Here's how the part is built. I have some questions about the finished solid (model axes, mm). A direction names the side the tool comes from. Coordinates: 2 decimals unless noted, no trailing zeros. Write each loop counter-clockwise with the first axis right and the second up, starting at its lowest first coordinate (ties: lowest second). Pieces come first, ordered by that corner, then holes. Notation, with made-up numbers: (35.25, 4.5) - (70.25, 4.5) arc R27 cw to (70.25, 41.5) - close; hole circle Ø6 at (-13.5, 63). An arc over 180 degrees is marked (long way). Answer in a Markdown table with one row per item. Add a question column.
Item 1: Imagine slicing it at C-C (z = 6.75). Please give me the cut outline in (x, y).
Item 2: Imagine slicing it at D-D (x = -4.5). Please give me the cut outline in (y, z), plus the area to 3 significant figures.
Item 3: Which directions (+Z, -Z, +X, -X, +Y, -Y) give clear straight access to the entire face, cutting with the end or side of a thin tool? Please do faces 1 (the face through (-5.5, 0, 1)), 2 (the face through (-0.3, 4.5, 0)), 3 (the face through (32, 0, 6)).
Item 4: If I drill on probe 1 along Y at (x, z) = (-15.9, 3); probe 2 along Y at (x, z) = (0, 2); probe 3 along Z at (x, y) = (4.5, 3.25), over which ranges is the centre line in solid material (lowest first)? Write a range as from..to.
Item 5: I'm going to push flat-ended pins straight in: pin 1 (3 mm diameter, centred on x = 17, y = 0.5, fed in from +Z); pin 2 (1 mm diameter, centred on y = 4, z = 3.5, fed in from -X). Where does each tip first touch, or does it pass through?
Item 6: Imagine slicing it at A-A (y = 0). State how many separate pieces and enclosed holes the cut face has, plus the area to 3 significant figures.
Item 7: We'd pull the mould along Y, two halves only. Please class faces 4 (the face through (-34.5, -0.1, 3)), 5 (the face through (-29, 0, 7.55)), 6 (the face through (5.5, 0, 1)), 7 (the face through (0, -5, 2)): +Y half, -Y half, draft (parallel to the pull), parting line (faces both ways), or undercut.
Item 8: Imagine slicing it at B-B (x = 15.9). Please give me the cut outline in (y, z).
Autodesk Inventor part; units mm, degrees
ref_plane "YZ Plane" through (0, 0, 0) normal (1, 0, 0) x (0, 1, 0)
ref_plane "XZ Plane" through (0, 0, 0) normal (0, 1, 0) x (-1, 0, 0)
ref_plane "XY Plane" through (0, 0, 0) normal (0, 0, 1) x (1, 0, 0)
sketch "Sketch1" plane through (0, 0, 0) normal (0, 0, 1) x (1, 0, 0)
  circle A0 centre (0, 0) radius 3
  circle A1 centre (0, 0) radius 5 construction
  circle A2 centre (-29.5, 0) radius 2.5
  circle A3 centre (29.5, 0) radius 2.5
  line L0 (-29.5, 0) -> (29.5, 0) construction
  arc A4 (-29.5, 5) -> (-29.5, -5) centre (-29.5, 0) ccw
  arc A5 (29.5, -5) -> (29.5, 5) centre (29.5, 0) ccw
  line L1 (-29.5, 5) -> (29.5, 5)
  line L2 (29.5, -5) -> (-29.5, -5)
  dimension "d0" = 6
  dimension "d1" = 10
  dimension "d2" = 5
  dimension "d3" = 5
  dimension "d4" = 29.5
  dimension "d5" = 29.5
  dimension "d6" = 2.5
  dimension "d7" = 2.5
extrude "Extrusion1" add sketch "Sketch1" along normal blind 4.05
sketch "Sketch2" plane through (0, 0, 0) normal (0, 0, -1) x (-1, 0, 0)
  line L0 (-5.5, -4) -> (5.5, -4)
  line L1 (5.5, -4) -> (5.5, 4)
  line L2 (5.5, 4) -> (-5.5, 4)
  line L3 (-5.5, 4) -> (-5.5, -4)
  line L4 (-5.5, -4) -> (5.5, 4) construction
  line L5 (5.5, -4) -> (-5.5, 4) construction
  line L6 (-29.5, 5) -> (29.5, 5)
  point P0 (0, 0)
  dimension "d10" = 8
  dimension "d11" = 11
extrude "Extrusion2" cut sketch "Sketch2" against normal blind 1.3
sketch "Sketch3" plane through (0, 0, 0) normal (0, 0, -1) x (-1, 0, 0)
  circle A0 centre (-29.5, 0) radius 2.5
  circle A1 centre (29.5, 0) radius 2.5
  point P0 (0, 0)
extrude "Extrusion3" add sketch "Sketch3" against normal blind 7.55
sketch "Sketch4" plane through (-29.5, 5, 0) normal (0, 1, 0) x (1, 0, 0)
  line L0 (64, 0) -> (64, -4.05)
  line L1 (64, -2) -> (64, 0)
  line L2 (59, 0) -> (64, 0)
  line L3 (64, 0) -> (48.5, 0)
  arc A0 (48.5, 0) -> (64, -2) centre (62.5699, 47.9795) ccw
  line L4 (59, 0) -> (0, 0)
  line L5 (29.5, 0) -> (29.5, -4.05)
  line L6 (59, -4.05) -> (0, -4.05)
  line L7 (-5, -2) -> (-5, 0)
  line L8 (0, 0) -> (-5, 0)
  line L9 (-5, 0) -> (10.5, 0)
  arc A1 (-5, -2) -> (10.5, 0) centre (-3.5699, 47.9795) ccw
  dimension "d16" = 19
  dimension "d17" = 2
  dimension "d18" = 50
extrude "Extrusion4" cut sketch "Sketch4" against normal through all
sketch "Sketch5" plane through (0, 0, 0) normal (0, 0, -1) x (-1, 0, 0)
  circle A0 centre (15.9, 0) radius 0.9
  circle A1 centre (-15.9, 0) radius 0.9
  line L0 (15.9, 0) -> (-15.9, 0)
  point P0 (0, 0)
  dimension "d21" = 1.8
  dimension "d22" = 1.8
  dimension "d24" = 15.9
extrude "Extrusion5" cut sketch "Sketch5" against normal through all
equation "\"d3\" = d2"
properties part number "gripper_mechanism1"
Here are the results:
| question | item | result |
|---|---|---|
| 1 | outline | circle Ø5 at (-29.5, 0); circle Ø5 at (29.5, 0) |
| 2 | outline | (-5, 0) - (-4, 0) - (-4, 1.3) - (4, 1.3) - (4, 0) - (5, 0) - (5, 4.05) - (-5, 4.05) - close |
| 2 | area | 30.1 mm2 |
| 3 | face 1 | -Z |
| 3 | face 2 | -Z, +X, -X, +Y, -Y |
| 3 | face 3 | +Z |
| 4 | probe 1 | y = -5..-0.9, 0.9..5 |
| 4 | probe 2 | y = -5..-3, 3..5 |
| 4 | probe 3 | z = 1.3..4.05 |
| 5 | pin 1 | stops at z = 4.05 |
| 5 | pin 2 | stops at x = -33.07 |
| 6 | separate pieces | 4 |
| 6 | enclosed holes | 0 |
| 6 | area | 225 mm2 |
| 7 | face 4 | parting line |
| 7 | face 5 | draft |
| 7 | face 6 | undercut |
| 7 | face 7 | -Y half |
| 8 | outline | (-5, 0) - (-0.9, 0) - (-0.9, 4.05) - (-5, 4.05) - close; (0.9, 0) - (5, 0) - (5, 4.05) - (0.9, 4.05) - close |
